```python
from build123d import *

# Parameters (mm, degrees)
DODANIE_WYCI_GNI_CIE1_DEPTH = 10
SZKIC5_R                    = 5.05
WYTNIJ_WYCI_GNI_CIE1_DEPTH  = 10
SZKIC9_R                    = 1.55
SZKIC9_W                    = 26
SZKIC9_H                    = 11
SZKIC9_W_2                  = 16
SZKIC9_H_2                  = 10
WYTNIJ_WYCI_GNI_CIE3_DEPTH  = 172.424567808
SZKIC13_R                   = 3.5
WYTNIJ_WYCI_GNI_CIE5_DEPTH  = 172.424567808
SZKIC19_W                   = 14.4
SZKIC19_H                   = 10.4
WYTNIJ_WYCI_GNI_CIE7_DEPTH  = 172.424567808
SZKIC20_R                   = 1.550000003
WYTNIJ_WYCI_GNI_CIE8_DEPTH  = 10
WYTNIJ_WYCI_GNI_CIE10_DEPTH = 10
WYTNIJ_WYCI_GNI_CIE11_DEPTH = 10
DODANIE_WYCI_GNI_CIE4_DEPTH = 10
SZKIC22_R                   = 1.55
WYTNIJ_WYCI_GNI_CIE9_DEPTH  = 10
WYTNIJ_WYCI_GNI_CIE6_DEPTH  = 172.424567808
WYTNIJ_WYCI_GNI_CIE12_DEPTH = 10
SZKIC30_R                   = 2.5
WYTNIJ_WYCI_GNI_CIE13_DEPTH = 10
WYTNIJ_WYCI_GNI_CIE14_DEPTH = 10


with BuildPart() as part:
    # Szkic2 → Dodanie-wyciągnięcie1 (new body)
    with BuildSketch(Plane(origin=(0, 0, 0), x_dir=(1, 0, 0), z_dir=(0, 1, 0))):
        with BuildLine():
            Line((-2.705874152, 127.916025413), (-8.705874152, 127.916025413))
            Line((-8.705874152, 127.916025413), (-8.722327105, 127.916025413))
            ThreePointArc((-8.722327105, 127.916025413), (-9.649740147, 127.688003136), (-10.365682355, 127.055930463))
            Line((-10.365682355, 127.055930463), (-32.779295153, 94.743126616))
            ThreePointArc((-32.779295153, 94.743126616), (-33.840904211, 92.57229607), (-34.205874152, 90.183506419))
            Line((-34.205874152, 90.183506419), (-34.205874152, -19.154356935))
            ThreePointArc((-34.205874152, -19.154356935), (-28.165753637, -33.476429577), (-13.693697675, -39.147797741))
            Line((-13.693697675, -39.147797741), (-2.713579886, -35.93445679))
            Line((-2.713579886, -35.93445679), (55.027168237, 21.545915465))
            ThreePointArc((55.027168237, 21.545915465), (56.334805154, 23.495770338), (56.794125848, 25.798132784))
            Line((56.794125848, 25.798132784), (56.794125848, 59.333926751))
            ThreePointArc((56.794125848, 59.333926751), (64.677605901, 81.048439594), (85.935948442, 90.090131813))
            Line((85.935948442, 90.090131813), (91.371133341, 90.090131813))
            ThreePointArc((91.371133341, 90.090131813), (105.458816444, 95.925441216), (111.294125848, 110.013124319))
            Line((111.294125848, 110.013124319), (111.294125848, 118.285035843))
            Line((111.294125848, 118.285035843), (111.294125848, 128))
            ThreePointArc((111.294125848, 128), (110.70833941, 129.414213562), (109.294125848, 130))
            Line((109.294125848, 130), (103.294125848, 130))
            ThreePointArc((103.294125848, 130), (101.879912285, 129.414213562), (101.294125848, 128))
            Line((101.294125848, 128), (101.294125848, 118.285035843))
            Line((101.294125848, 118.285035843), (101.294125848, 110))
            ThreePointArc((101.294125848, 110), (98.36519366, 102.928932188), (91.294125848, 100))
            Line((91.294125848, 100), (9.294125848, 100))
            ThreePointArc((9.294125848, 100), (2.223058036, 102.928932188), (-0.705874152, 110))
            Line((-0.705874152, 110), (-0.705874152, 125.916025413))
            ThreePointArc((-0.705874152, 125.916025413), (-1.291660589, 127.330238976), (-2.705874152, 127.916025413))
        make_face()
    extrude(amount=DODANIE_WYCI_GNI_CIE1_DEPTH)

    # Szkic5 → Wytnij-wyciągnięcie1 (cut)
    with BuildSketch(Plane(origin=(0, 10, 0), x_dir=(1, 0, 0), z_dir=(0, 1, 0))):
        with Locations(Location((-13.29618586, -25.303913492, 0), (0, 0, 270))):
            Circle(SZKIC5_R)
    extrude(amount=-WYTNIJ_WYCI_GNI_CIE1_DEPTH, mode=Mode.SUBTRACT)

    # Szkic9 → Wytnij-wyciągnięcie3 (cut, through all)
    with BuildSketch(Plane(origin=(0, 10, 0), x_dir=(1, 0, 0), z_dir=(0, 1, 0))):
        with Locations(Location((17.894125848, 72, 0), (0, 0, 270))):
            Circle(SZKIC9_R)
        with Locations((10.894125848, 52.5)):
            Rectangle(SZKIC9_W, SZKIC9_H)
        with Locations((15.894125848, 85)):
            Rectangle(SZKIC9_W_2, SZKIC9_H_2)
    extrude(amount=-WYTNIJ_WYCI_GNI_CIE3_DEPTH, mode=Mode.SUBTRACT)

    # Szkic13 → Wytnij-wyciągnięcie5 (cut, through all)
    with BuildSketch(Plane(origin=(0, 10, 0), x_dir=(1, 0, 0), z_dir=(0, 1, 0))):
        with Locations(Location((40.894125848, 75.45, 0), (0, 0, 270))):
            Circle(SZKIC13_R)
        with Locations(Location((40.894125848, 46.55, 0), (0, 0, 270))):
            Circle(SZKIC13_R)
        with Locations(Location((30.260526653, 95, 0), (0, 0, 270))):
            Circle(SZKIC13_R)
        with Locations(Location((6.36054282, 95, 0), (0, 0, 270))):
            Circle(SZKIC13_R)
    extrude(amount=-WYTNIJ_WYCI_GNI_CIE5_DEPTH, mode=Mode.SUBTRACT)

    # Szkic19 → Wytnij-wyciągnięcie7 (cut, through all)
    with BuildSketch(Plane(origin=(0, 10, 0), x_dir=(1, 0, 0), z_dir=(0, 1, 0))):
        with Locations((-19.205874152, 93.746086503)):
            Rectangle(SZKIC19_W, SZKIC19_H)
    extrude(amount=-WYTNIJ_WYCI_GNI_CIE7_DEPTH, mode=Mode.SUBTRACT)

    # Szkic20 → Wytnij-wyciągnięcie8 (cut)
    with BuildSketch(Plane.XZ):
        with Locations(Location((-29.337186678, -72.387878862, 0), (0, 0, 270))):
            Circle(SZKIC20_R)
    extrude(amount=-WYTNIJ_WYCI_GNI_CIE8_DEPTH, mode=Mode.SUBTRACT)

    # Szkic23 → Wytnij-wyciągnięcie10 (cut)
    with BuildSketch(Plane(origin=(0, 10, 0), x_dir=(1, 0, 0), z_dir=(0, 1, 0))):
        with BuildLine():
            Line((15.628724602, 38.350669498), (8.597420665, 21.889479841))
            Line((8.597420665, 21.889479841), (-0.782698582, 25.896144654))
            Line((-0.782698582, 25.896144654), (6.248605356, 42.357334312))
            ThreePointArc((6.248605356, 42.357334312), (12.941997386, 45.044061528), (15.628724602, 38.350669498))
        make_face()
    extrude(amount=-WYTNIJ_WYCI_GNI_CIE10_DEPTH, mode=Mode.SUBTRACT)

    # Szkic25 → Wytnij-wyciągnięcie11 (cut)
    with BuildSketch(Plane(origin=(0, 10, 0), x_dir=(1, 0, 0), z_dir=(0, 1, 0))):
        with BuildLine():
            Line((1.679385524, 31.66020119), (3.469714538, 35.85159239))
            Line((3.469714538, 35.85159239), (3.704708682, 36.109613041))
            ThreePointArc((3.704708682, 36.109613041), (9.518980065, 39.386499344), (13.410780858, 33.964541935))
            Line((13.410780858, 33.964541935), (13.39199801, 33.114203976))
            Line((13.39199801, 33.114203976), (12.051775457, 29.976570072))
            Line((12.051775457, 29.976570072), (11.05950477, 27.653536376))
            Line((11.05950477, 27.653536376), (17.589964961, -6.167500607))
            ThreePointArc((17.589964961, -6.167500607), (13.061179445, -14.403704543), (4.044681841, -11.748949479))
            ThreePointArc((4.044681841, -11.748949479), (-4.827370085, -4.988355381), (-15.874459375, -3.445385461))
            ThreePointArc((-15.874459375, -3.445385461), (-23.818044234, 0.469833912), (-22.492396316, 9.226096856))
            Line((-22.492396316, 9.226096856), (1.679385524, 31.66020119))
        make_face()
    extrude(amount=-WYTNIJ_WYCI_GNI_CIE11_DEPTH, mode=Mode.SUBTRACT)

    # Szkic27 → Dodanie-wyciągnięcie4 (add)
    with BuildSketch(Plane.XZ):
        with BuildLine():
            Line((111.294125848, -110.013124319), (91.371133341, -90.090131813))
            Line((91.371133341, -90.090131813), (85.935948442, -90.090131813))
            ThreePointArc((85.935948442, -90.090131813), (64.677605901, -81.048439594), (56.794125848, -59.333926751))
            Line((56.794125848, -59.333926751), (56.794125848, -25.798132784))
            Line((56.794125848, -25.798132784), (55.027168237, -21.545915465))
            Line((55.027168237, -21.545915465), (-2.713579886, 35.93445679))
            Line((-2.713579886, 35.93445679), (-13.693697675, 39.147797741))
            Line((-13.693697675, 39.147797741), (7.831109821, 38.596391899))
            ThreePointArc((7.831109821, 38.596391899), (16.200857661, 35.992910672), (22.653502952, 30.060443886))
            Line((22.653502952, 30.060443886), (62.775344571, -27.781601032))
            Line((62.775344571, -27.781601032), (89.166132073, -65.828137643))
            Line((89.166132073, -65.828137643), (107.72767835, -92.58757216))
            ThreePointArc((107.72767835, -92.58757216), (110.381700996, -98.014648527), (111.294125848, -103.986622655))
            Line((111.294125848, -103.986622655), (111.294125848, -110.013124319))
        make_face()
    extrude(amount=-DODANIE_WYCI_GNI_CIE4_DEPTH)

    # Szkic22 → Wytnij-wyciągnięcie9 (cut)
    with BuildSketch(Plane.XZ):
        with Locations(Location((63.668699874, -36.964909883, 0), (0, 0, 270))):
            Circle(SZKIC22_R)
    extrude(amount=-WYTNIJ_WYCI_GNI_CIE9_DEPTH, mode=Mode.SUBTRACT)

    # Szkic17 → Wytnij-wyciągnięcie6 (cut, through all)
    with BuildSketch(Plane(origin=(0, 10, 0), x_dir=(1, 0, 0), z_dir=(0, 1, 0))):
        Polygon((66.124221849, 58.029118396), (78.203911754, 71.908638986), (70.358965334, 78.736289802), (58.279275429, 64.856769212), align=None)
    extrude(amount=-WYTNIJ_WYCI_GNI_CIE6_DEPTH, mode=Mode.SUBTRACT)

    # Szkic28 → Wytnij-wyciągnięcie12 (cut)
    with BuildSketch(Plane(origin=(0, 10, 0), x_dir=(1, 0, 0), z_dir=(0, 1, 0))):
        with BuildLine():
            Line((11.26748333, 26.576422306), (10.066738772, 23.271111531))
            Line((10.066738772, 23.271111531), (13.650053515, 4.713243184))
            Line((13.650053515, 4.713243184), (14.443246416, -0.151068703))
            Line((14.443246416, -0.151068703), (16.401806069, -0.01406507))
            ThreePointArc((16.401806069, -0.01406507), (16.908780733, 1.735462564), (18.624084966, 2.348326041))
            ThreePointArc((18.624084966, 2.348326041), (19.396162916, 2.285491306), (20.170698513, 2.297622868))
            Line((20.170698513, 2.297622868), (20.24930544, 2.302668096))
            ThreePointArc((20.24930544, 2.302668096), (23.123159184, 3.803925799), (23.940405993, 6.941586981))
            Line((23.940405993, 6.941586981), (23.056429184, 12.118910521))
            Line((23.056429184, 12.118910521), (22.000864003, 18.666304586))
            ThreePointArc((22.000864003, 18.666304586), (20.623069051, 21.574602066), (17.93652414, 23.346321457))
            Line((17.93652414, 23.346321457), (12.620467249, 25.051129714))
            ThreePointArc((12.620467249, 25.051129714), (11.735014139, 25.628420704), (11.26748333, 26.576422306))
        make_face()
        with BuildLine():
            Line((-0.358990635, 31.193922826), (-5.655504297, 32.95851204))
            ThreePointArc((-5.655504297, 32.95851204), (-8.869808875, 33.115862726), (-11.699467807, 31.583040659))
            Line((-11.699467807, 31.583040659), (-13.721552832, 29.619702325))
            Line((-13.721552832, 29.619702325), (-20.075654798, 23.596300827))
            ThreePointArc((-20.075654798, 23.596300827), (-21.322767717, 20.6033893), (-19.942342747, 17.669580012))
            Line((-19.942342747, 17.669580012), (-19.882798357, 17.618014821))
            ThreePointArc((-19.882798357, 17.618014821), (-19.179679353, 17.074421967), (-18.420602931, 16.612174728))
            ThreePointArc((-18.420602931, 16.612174728), (-17.380074633, 15.099249316), (-18.012101151, 13.375246728))
            Line((-18.012101151, 13.375246728), (-18.878230506, 12.580445054))
            Line((-18.878230506, 12.580445054), (-17.460533124, 11.447059157))
            Line((-17.460533124, 11.447059157), (-13.203312435, 15.39161053))
            Line((-13.203312435, 15.39161053), (0.650139771, 28.249156335))
            Line((0.650139771, 28.249156335), (1.63370973, 31.625464518))
            ThreePointArc((1.63370973, 31.625464518), (0.696479646, 31.136698863), (-0.358990635, 31.193922826))
        make_face()
    extrude(amount=-WYTNIJ_WYCI_GNI_CIE12_DEPTH, mode=Mode.SUBTRACT)

    # Szkic30 → Wytnij-wyciągnięcie13 (cut)
    with BuildSketch(Plane.XZ):
        with Locations(Location((50.565790387, -80.001305931, 0), (0, 0, 270))):
            Circle(SZKIC30_R)
        with Locations(Location((50.48451947, -95.001085764, 0), (0, 0, 270))):
            Circle(SZKIC30_R)
    extrude(amount=-WYTNIJ_WYCI_GNI_CIE13_DEPTH, mode=Mode.SUBTRACT)

    # Szkic31 → Wytnij-wyciągnięcie14 (cut)
    with BuildSketch(Plane.XZ):
        with BuildLine():
            Line((14.621138887, 30.235921356), (57.465724426, -31.531393932))
            ThreePointArc((57.465724426, -31.531393932), (59.396767725, -32.773629705), (61.640614875, -32.286569233))
            Line((61.640614875, -32.286569233), (62.051453688, -32.00159297))
            ThreePointArc((62.051453688, -32.00159297), (64.295300838, -31.514532498), (66.226344137, -32.756768271))
            Line((66.226344137, -32.756768271), (22.653502952, 30.060443886))
            ThreePointArc((22.653502952, 30.060443886), (16.200857661, 35.992910672), (7.831109821, 38.596391899))
            Line((7.831109821, 38.596391899), (-1.300237138, 38.830311667))
            ThreePointArc((-1.300237138, 38.830311667), (7.687866321, 36.436435661), (14.621138887, 30.235921356))
        make_face()
    extrude(amount=-WYTNIJ_WYCI_GNI_CIE14_DEPTH, mode=Mode.SUBTRACT)


solid = part.part
```
Geometry: final body of the model. Coordinates: model frame, mm. A direction names the side the tool comes from. Round coordinates to 2 decimals unless told otherwise and drop trailing zeros. Write each loop counter-clockwise with the first axis right and the second up, starting at its lowest first coordinate (ties: lowest second). Pieces come first, ordered by that corner, then holes.
Item 1: Pin query (flat end, axial travel): P1, Ø6.5, axis at x = 40.89, z = -46.55, coming from the +Y side; P2, Ø3, axis at y = 2.5, z = -94.5, coming from the +X side; P3, Ø3, axis at y = 6, z = -94, coming from the +X side; P4, Ø3, axis at x = 19.5, y = 3.5, coming from the +Z side. Return the tip coordinate at first contact, or that it passes through.
Item 2: Material intervals for L1, parallel to Z at x = 49, y = 3.25; L2, parallel to X at y = 8, z = -81.5; L3, parallel to Z at x = 42.5, y = 9, sorted ascending.
Item 3: Section query A-A (z = -116.5). Return loops of the section in (x, y).
Item 4: Set-up query: faces 5 (the face through (16, 5, -80)), 6 (the face through (101.294, 5, -119)), 7 (the face through (-6, 5, -127.916)). Return all of +Z, -Z, +X, -X, +Y, -Y with unobstructed straight access to the full face (end or side cutting, diameter ignored); none if empty.
Item 5: Section query B-B (y = 3). Give the number of separate pieces and of enclosed holes in the cut face, plus the area to 3 significant figures.
Item 6: Mould query, pull axis Z, two halves, no side actions, for faces 1 (the face through (59.364, 4.93, -32.768)), 2 (the face through (64.4, 5.07, -71.89)), 3 (the face through (21.4, 0, -46.6)), 4 (the face through (-21.416, 4.93, -111.126)). Classes: +Z half, -Z half, draft (parallel to the pull), parting line (faces both ways), or undercut.
Item 7: Section query C-C (x = 97). Return loops of the section in (y, z).
Completed:
1. P1: passes through
1. P2: stops at x = 109.63
1. P3: stops at x = 109.4
1. P4: stops at z = 25.36
2. L1: z = -100 to -97.01, -92.99 to -81.95, -78.05 to -19.33
2. L2: x = -34.21 to 7.89, 23.89 to 48.56, 52.57 to 100.04
2. L3: z = -100 to -78.56, -72.34 to -49.66, -43.44 to -9.96
3. outline: (-17.69, 0) - (-0.71, 0) - (-0.71, 10) - (-17.69, 10) - close; (101.29, 0) - (111.29, 0) - (111.29, 10) - (101.29, 10) - close
4. face 5: +Y, -Y
4. face 6: -Z, +Y, -Y
4. face 7: -Z, -X, +Y, -Y
5. separate pieces: 1
5. enclosed holes: 15
5. area: 11,100 mm2
6. face 1: +Z half
6. face 2: undercut
6. face 3: draft
6. face 4: -Z half
7. outline: (0, -101.79) - (10, -101.79) - (10, -77.12) - (0, -77.12) - close
